Check sheet for the modelled part. Datum: model origin and axes. Units: mm. A direction names the side the tool comes from. Coordinates: 2 decimals unless noted, no trailing zeros. Loops run counter-clockwise (first coordinate to the right, second up) from the corner with the lowest first, then second, coordinate; pieces in that order, holes last. Notation, with made-up numbers: M 74.25,-1 L 86.25,-1 A21 ccw 86.25,26 Z; hole C 35.5,74 d6. An arc over 180 degrees is marked long. Answer as CSV lines item,"result". Start each with the question number.
from build123d import *

# Parameters (mm, degrees)
BOSS_EXTRUDE1_DEPTH = 15
SKETCH2_R           = 2.625
CUT_EXTRUDE1_DEPTH  = 16
SKETCH3_R           = 12.2
CUT_EXTRUDE2_DEPTH  = 20
CUT_EXTRUDE5_DEPTH  = 10
SKETCH6_W           = 14
SKETCH6_H           = 20
SKETCH6_W_2         = 20
SKETCH6_H_2         = 14
CUT_EXTRUDE6_DEPTH  = 10
SKETCH8_W           = 10
SKETCH8_H           = 5
SKETCH8_W_2         = 5
SKETCH8_H_2         = 10
CUT_EXTRUDE7_DEPTH  = 5


with BuildPart() as part:
    # Sketch1 → Boss-Extrude1 (new body)
    with BuildSketch(Plane.XY):
        with BuildLine():
            Line((0, 100), (0, 0))
            Line((0, 0), (-100, 0))
            ThreePointArc((-100, 0), (-70.710678118, 70.710678118), (0, 100))
        make_face()
    extrude(amount=BOSS_EXTRUDE1_DEPTH)

    # Sketch2 → Cut-Extrude1 (cut, through all)
    with BuildSketch(Plane.XY):
        with Locations((-7.76457135, 28.97777479)):
            Circle(SKETCH2_R)
        with Locations((-21.213203434, 21.213203438)):
            Circle(SKETCH2_R)
        with Locations((-28.977774788, 7.764571356)):
            Circle(SKETCH2_R)
    extrude(amount=CUT_EXTRUDE1_DEPTH, mode=Mode.SUBTRACT)

    # Sketch3 → Cut-Extrude2 (cut)
    with BuildSketch(Plane.XY):
        Circle(SKETCH3_R)
    extrude(amount=CUT_EXTRUDE2_DEPTH, mode=Mode.SUBTRACT)

    # Sketch5 → Cut-Extrude5 (cut)
    with BuildSketch(Plane.XY):
        Polygon((-71.95873614, 20.826742868), (-61.115668074, 11.728328454), (-14.639983633, 67.115892355), (-25.483051698, 76.21430677), align=None)
        Polygon((-58.563247101, 10.460640314), (-47.720179035, 1.3622259), (-1.244494594, 56.749789802), (-12.087562659, 65.848204216), align=None)
        Polygon((-85.713169601, 31.896516461), (-74.870101536, 22.798102046), (-28.394417094, 78.185665948), (-39.237485159, 87.284080363), align=None)
    extrude(amount=CUT_EXTRUDE5_DEPTH, mode=Mode.SUBTRACT)

    # Sketch6 → Cut-Extrude6 (cut)
    with BuildSketch(Plane.XY):
        with Locations((-9.9593736, 84.419453757)):
            Rectangle(SKETCH6_W, SKETCH6_H)
        with Locations((-83.670510765, 9.900506549)):
            Rectangle(SKETCH6_W_2, SKETCH6_H_2)
    extrude(amount=CUT_EXTRUDE6_DEPTH, mode=Mode.SUBTRACT)

    # Sketch8 → Cut-Extrude7 (cut)
    with BuildSketch(Plane.XY):
        Polygon((-43.599799459, 8.831466661), (-89.403952996, 46.904961374), (-92.064810722, 42.671778628), (-46.260657185, 4.598283915), align=None)
        with Locations((-96.259669563, 9.424871496)):
            Rectangle(SKETCH8_W, SKETCH8_H)
        with Locations((-10.06190419, 97.056119442)):
            Rectangle(SKETCH8_W_2, SKETCH8_H_2)
    extrude(amount=CUT_EXTRUDE7_DEPTH, mode=Mode.SUBTRACT)


solid = part.part
Item 1: Sectioned sample at C-C, the plane x = -63.5. Record the boundary of the cut face in (y, z).
Item 2: Set-up check for faces 5 (the face through (-10, 97, 5)), 6 (the face through (-97, 6.925, 2)), 7 (the face through (-10, 85, 10)): record each of +Z, -Z, +X, -X, +Y, -Y from which the full face is reachable in a straight line by a thin tool's end or side.
Item 3: Material ranges on line 1 (X direction, y = 8.5, z = 2); line 2 (Y direction, x = -11, z = 9); line 3 (Y direction, x = -41, z = 9.25), recorded low to high. Write a range as from..to.
Item 4: Go/stop test with flat-tipped pins: pin 1 (3 mm diameter, centred on x = -6.5, z = 6, fed in from -Y); pin 2 (2.5 mm diameter, centred on x = -56, y = 16, fed in from -Z); pin 3 (4.5 mm diameter, centred on x = -7.76, y = 28.98, fed in from +Z); pin 4 (8 mm diameter, centred on y = 79.5, z = 4, fed in from -X). Record where each tip stops, or that it passes through.
Item 5: Sectioned sample at A-A, the plane z = 12. Record the boundary of the cut face in (x, y) (3 decimals).
Item 6: Sectioned sample at D-D, the plane y = 61. Record the boundary of the cut face in (x, z).
Item 7: Sectioned sample at B-B, the plane y = 50. Record the boundary of the cut face in (x, z) (3 decimals).
Item 8: Release check for a two-part mould opening along Y. For faces 1 (the face through (-55, 0, 7)), 2 (the face through (-2.959, 84, 5)), 3 (the face through (-84, 2.901, 5)), 4 (the face through (-71.484, 69.929, 7.395)) record: released by +Y, released by -Y, zero draft, split by the parting line, or undercut.
Reply:
1,outline,"M 0,0 L 13.73,0 L 13.73,10 L 30.91,10 L 30.91,0 L 36.35,0 L 36.35,10 L 58.37,10 L 58.37,0 L 77.25,0 L 77.25,15 L 0,15 Z"
2,face 5,"-Z, +Y"
2,face 6,"-Z, -X"
2,face 7,"-Z"
3,line 1,"-73.67..-56.23, -41.73..-31.5, -26.46..-8.75"
3,line 2,"5.28..45.12, 64.94..74.42, 94.42..99.39"
3,line 3,"0..9.37, 31.39..35.7, 57.72..63.16, 85.18..91.21"
4,pin 1,"y = 9.21"
4,pin 2,"z = 5"
4,pin 3,"through"
4,pin 4,"x = -65.57"
5,outline,"M -100,0 L -12.2,0 A12.2 cw 0,12.2 L 0,100 A100 ccw Z; hole C -28.978,7.765 d5.25; hole C -21.213,21.213 d5.25; hole C -7.765,28.978 d5.25"
6,outline,"M -79.24,0 L -61.29,0 L -61.29,10 L -42.81,10 L -42.81,0 L -38.25,0 L -38.25,10 L -19.77,10 L -19.77,0 L -16.16,0 L -16.16,10 L -6.31,10 L -6.31,0 L 0,0 L 0,15 L -79.24,15 Z"
7,outline,"M -86.603,0 L -70.523,0 L -70.523,10 L -52.045,10 L -52.045,0 L -47.479,0 L -47.479,10 L -29.002,10 L -29.002,0 L -25.386,0 L -25.386,10 L -6.908,10 L -6.908,0 L 0,0 L 0,15 L -86.603,15 Z"
8,face 1,"released by -Y"
8,face 2,"undercut"
8,face 3,"undercut"
8,face 4,"released by +Y"
